from build123d import *

# Parameters (mm, degrees)
F0_W     = 1828.8
F0_H     = 88.9
F0_W_2   = 38.1
F0_H_2   = 25.4
F0_R     = 31.75
F1_DEPTH = 19.05


with BuildPart() as f1:
    # F0 (on Front) → F1 (new body)
    with BuildSketch(Plane.XZ):
        Rectangle(F0_W, F0_H)
        with Locations((-777.044298, -12.7)):
            Rectangle(F0_W_2, F0_H_2, mode=Mode.SUBTRACT)
        with Locations((739.726365, -13.886383)):
            Rectangle(F0_W_2, F0_H_2, mode=Mode.SUBTRACT)
        with Locations((-316.060573, 0)):
            Circle(F0_R, mode=Mode.SUBTRACT)
        with Locations((328.7251, 0)):
            Circle(F0_R, mode=Mode.SUBTRACT)
    extrude(amount=F1_DEPTH)


solid = f1.part
Geometry: final body of the model. Coordinates: model frame, mm. Give positions to 0.01 mm unless a question says otherwise; leave off trailing zeros. Write each loop counter-clockwise with the first axis right and the second up, starting at its lowest first coordinate (ties: lowest second). Pieces come first, ordered by that corner, then holes. Notation, with made-up numbers: M 20.5,62 L 72.5,62 A21 cw 72.5,84 Z; hole C 63,54 d9. An arc over 180 degrees is marked long. Answer in a Markdown table with one row per item. Add a question column.
(1) Ray query, line 1 (X direction, y = -3.25, z = -25.5); line 2 (X direction, y = -15.25, z = -26); line 3 (X direction, y = -17.5, z = 28). Return the intervals inside material, ascending.
(2) Section A-A on y = -8.75. Return loops of the section in (x, z).
(3) Mould query, pull axis X, two halves, no side actions, for faces 1 (the cylindrical face through (359.01, -9.39, 9.54)), 2 (the flat face through (-13, 0, 1)), 3 (the cylindrical face through (-285.777, -9.392, 9.537)). Classes: +X half, -X half, draft (parallel to the pull), parting line (faces both ways), or undercut.
(4) First-contact query: pin 1 (1.5 mm diameter, centred on x = -449.5, z = -25.5, fed in from +Y). Flat tip, straight axial feed; report the tip coordinate or a pass-through.
Result set:
| question | item | result |
|---|---|---|
| 1 | line 1 | x = -914.4 to -334.98, -297.14 to 309.81, 347.64 to 720.68, 758.78 to 914.4 |
| 1 | line 2 | x = -914.4 to -334.28, -297.84 to 310.5, 346.95 to 720.68, 758.78 to 914.4 |
| 1 | line 3 | x = -914.4 to -331.03, -301.09 to 313.76, 343.69 to 914.4 |
| 2 | outline | M -914.4,-44.45 L 914.4,-44.45 L 914.4,44.45 L -914.4,44.45 Z; hole M -796.09,-25.4 L -757.99,-25.4 L -757.99,0 L -796.09,0 Z; hole C -316.06,0 d63.5; hole C 328.73,0 d63.5; hole M 720.68,-26.59 L 758.78,-26.59 L 758.78,-1.19 L 720.68,-1.19 Z |
| 3 | face 1 | undercut |
| 3 | face 2 | draft |
| 3 | face 3 | undercut |
| 4 | pin 1 | stops at y = 0 |
